Can you work these out from the model? Positions are in its coordinate system, mm. A direction names the side the tool comes from. Coordinates: 2 decimals unless noted, no trailing zeros. Order: outer loops, then holes, each group sorted by start corner. A loop starts at its lowest first (then second) coordinate and runs counter-clockwise, first axis right, second up. Notation, with made-up numbers: (13.25, 73) -> (23.25, 73) arc R21 cw to (23.25, 104) -> close; hole circle Ø5 at (80.25, 32.5). An arc over 180 degrees is marked (long way). Return JSON: item names as keys, results as strings. Group by question number.
1) For faces 1 (the flat face through (0, 32, 15)), 2 (the flat face through (0, 32, -15)), 3 (the flat face through (15, 32, 0)), which set-ups out of +Z, -Z, +X, -X, +Y, -Y let a thin tool reach every point of the face, with its end or its side?
2) For pin 1 (3 mm diameter, centred on x = 6, y = 7.5, fed in from -Z); pin 2 (5 mm diameter, centred on x = 15.5, z = 16, fed in from -Y); pin 3 (4 mm diameter, centred on x = 19, z = -10, fed in from -Y), each with a flat end and sliding along its axis, tell me the tip position at first contact or that it passes through.
3) If we section it at B-B, the plane z = -5: Please give me the cut outline in (x, y).
4) If we section it at D-D, the plane x = 0: Please give me the cut outline in (y, z), then the cut area to 3 significant figures.
5) If I drill on probe 1 along Y at (x, z) = (11.5, 16.5); probe 2 along Z at (x, y) = (-2.5, 9); probe 3 along Y at (x, z) = (0.5, -12.5), over which ranges is the centre line in solid material (lowest first)? Write a range as from..to.
6) If we section it at A-A, the plane x = 20: Please give me the cut outline in (y, z).
7) If we section it at C-C, the plane y = 30.5: Please give me the cut outline in (x, z).
8) Thinking about a two-plate mould opening in Y: for faces 4 (the flat face through (0, 20, 13)), 5 (the flat face through (-15, 32, 0)), 6 (the flat face through (0, -3, -10)), which applies, +Y half, -Y half, draft (parallel to the pull), parting line (faces both ways), or undercut?
from build123d import *

# Parameters (mm, degrees)
SK_CASTERWHEEL_W = 25
SK_CASTERWHEEL_H = 20
SK_FORK_W        = 30
SK_FORK_H        = 24
FORK_DEPTH       = 15
SK_TOPPLATE_W    = 50
SK_TOPPLATE_H    = 3
TOPPLATE_DEPTH   = 20


with BuildPart() as part:
    # SK_CasterWheel → CasterWheel (revolve)
    with BuildSketch(Plane(origin=(0, 0, 0), x_dir=(1, 0, 0), z_dir=(0, 1, 0)), mode=Mode.PRIVATE) as casterwheel_sk:
        with Locations((12.5, 0)):
            Rectangle(SK_CASTERWHEEL_W, SK_CASTERWHEEL_H)
    revolve(casterwheel_sk.sketch.rotate(Axis((0, 0, -15), (0, 0, 1)), 180), axis=Axis((0, 0, -15), (0, 0, 1)))

    # SK_Fork → Fork (add, symmetric)
    with BuildSketch(Plane.XY):
        with Locations((0, 32)):
            Rectangle(SK_FORK_W, SK_FORK_H)
    extrude(amount=FORK_DEPTH, both=True)

    # SK_TopPlate → TopPlate (add, symmetric)
    with BuildSketch(Plane.XY):
        with Locations((0, 45.5)):
            Rectangle(SK_TOPPLATE_W, SK_TOPPLATE_H)
    extrude(amount=TOPPLATE_DEPTH, both=True)


solid = part.part
Result sheet:
{
 "1": {"face 1": "+Z, +X, -X, -Y", "face 2": "-Z, +X, -X, -Y", "face 3": "+Z, -Z, +X"},
 "2": {"pin 1": "stops at z = -10", "pin 2": "stops at y = 20", "pin 3": "stops at y = -18.33"},
 "3": {"outline": "(-25, 44) -> (-15, 44) -> (-15, 20) arc R25 ccw (long way) to (15, 20) -> (15, 44) -> (25, 44) -> (25, 47) -> (-25, 47) -> close"},
 "4": {"outline": "(-25, -10) -> (20, -10) -> (20, -15) -> (44, -15) -> (44, -20) -> (47, -20) -> (47, 20) -> (44, 20) -> (44, 15) -> (20, 15) -> (20, 10) -> (-25, 10) -> close", "area": "1,740 mm2"},
 "5": {"probe 1": "y = 44..47", "probe 2": "z = -10..10", "probe 3": "y = 20..47"},
 "6": {"outline": "(-15, -10) -> (15, -10) -> (15, 10) -> (-15, 10) -> close; (44, -20) -> (47, -20) -> (47, 20) -> (44, 20) -> close"},
 "7": {"outline": "(-15, -15) -> (15, -15) -> (15, 15) -> (-15, 15) -> close"},
 "8": {"face 4": "-Y half", "face 5": "undercut", "face 6": "draft"}
}
